Design review of the part shown in the three views and the two pictorial views. Dimensions are in mm from the part's minimum x, y and z. Coordinates: 2 decimals unless noted, no trailing zeros. Loops run counter-clockwise (first coordinate to the right, second up) from the corner with the lowest first, then second, coordinate; pieces in that order, holes last. Notation, with made-up numbers: (80.5, 77.25) - (107.5, 77.25) arc R22 cw to (107.5, 88.25) - close; hole circle Ø11 at (69, -4). An arc over 180 degrees is marked (long way). One line per question, with ' | ' between items.
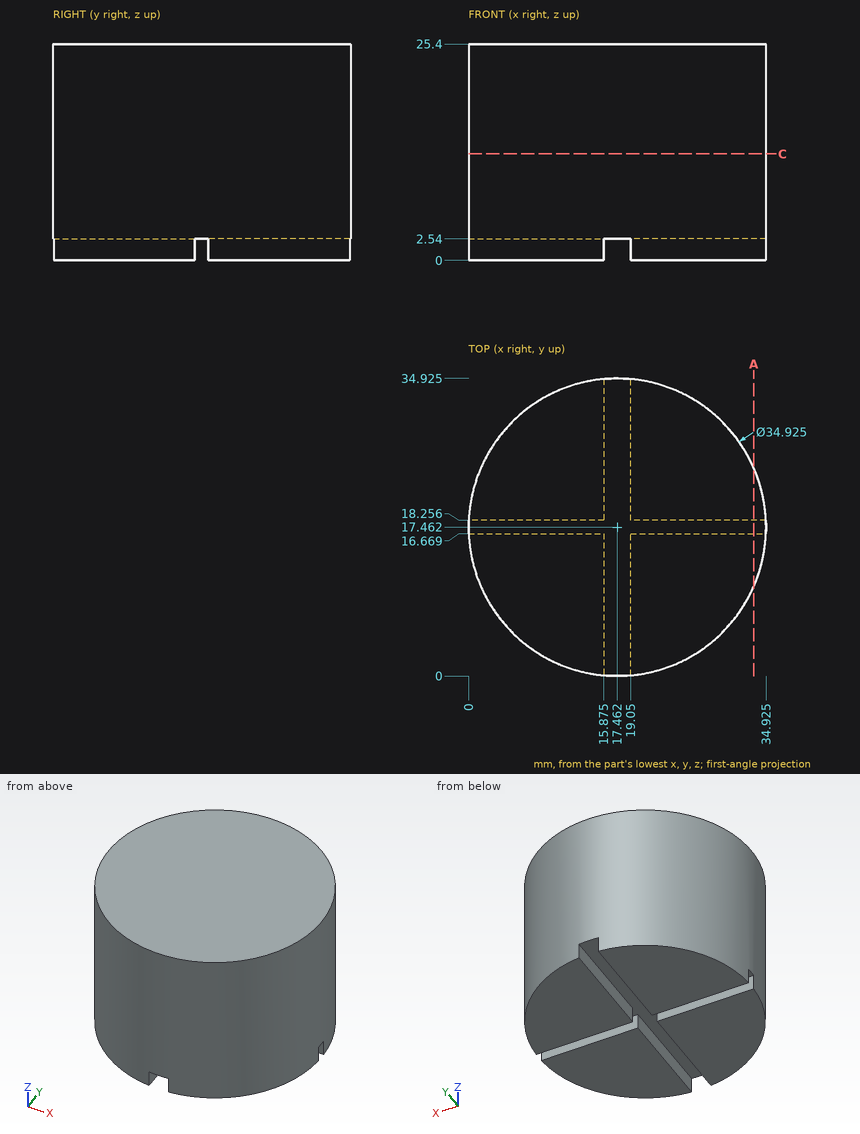
Q1. To check wall thickness, follow line 1 along Z through (x, y) = (18.5, 2.5); line 2 along Y through (x, z) = (26.5, 2.5) (1 decimal); line 3 along X through (y, z) = (13, 17.5) (1 decimal). State the ranges of each line that lie inside material, in increasing order.
Returned:
line 1: z = 2.54 to 25.4 | line 2: y = 2.5 to 16.7, 18.3 to 32.4 | line 3: x = 0.6 to 34.3
Q2. For pin 1 (1.3 mm diameter, centred on x = 11, z = 1, fed in from +Y); pin 2 (3 mm diameter, centred on y = 24.5, z = 1.5, fed in from +X); pin 3 (1.3 mm diameter, centred on y = 25, z = 1.5, fed in from -X) (1 decimal), all flat-tipped, find the tip position at first contact; note any pin that passes through.
Returned:
pin 1: stops at y = 33.93 | pin 2: stops at x = 34.02 | pin 3: stops at x = 1.4
Q3. Take a section at A-A (x = 33.5). Give the boundary of the cut face in (y, z), plus the area to 3 significant figures.
Returned:
outline: (10.55, 0) - (16.67, 0) - (16.67, 2.54) - (18.26, 2.54) - (18.26, 0) - (24.37, 0) - (24.37, 25.4) - (10.55, 25.4) - close | area: 347 mm²
Q4. Take a section at C-C (z = 12.5). Give the boundary of the cut face in (x, y) (1 decimal).
Returned:
outline: circle Ø34.9 at (17.5, 17.5)
